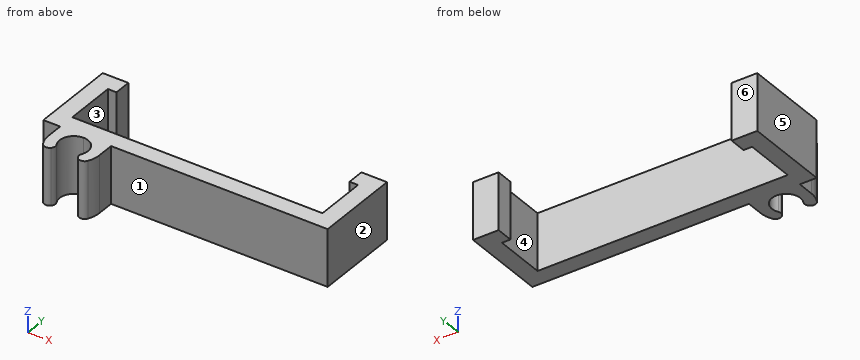
```python
from build123d import *

# Parameters (mm, degrees)
F1_DEPTH    = 10
F2_T1_DEPTH = 16.5073043021
F2_T3_DEPTH = 14.2705098312


# Not quite as in the source:
# - a fillet or chamfer that OpenCascade refuses, or shapes differently, is made with other operations: its cross-section is extruded or revolved along the edge and cut away or added


with BuildPart() as f1:
    # F0 (on Top) → F1 (new body)
    with BuildSketch(Plane.XY):
        with BuildLine():
            Line((-25.6786430255, 0), (12.4131741374, 0))
            Line((12.4131741374, 0), (12.4131741374, 15))
            Line((12.4131741374, 15), (7.9131741374, 15))
            Line((7.9131741374, 15), (7.9131741374, 12))
            Line((7.9131741374, 12), (9.4131741374, 12))
            Line((9.4131741374, 12), (9.4131741374, 3))
            Line((9.4131741374, 3), (-34.5868258626, 3))
            Line((-34.5868258626, 3), (-34.5868258626, 12))
            Line((-34.5868258626, 12), (-33.0868258626, 12))
            Line((-33.0868258626, 12), (-33.0868258626, 15))
            Line((-33.0868258626, 15), (-37.5868258626, 15))
            Line((-37.5868258626, 15), (-37.5868258626, 0))
            Line((-37.5868258626, 0), (-34.6318436787, 0))
            Line((-34.6318436787, 0), (-34.6318436787, -2.9766003136))
            ThreePointArc((-34.6318436787, -2.9766003136), (-34.291082769, -4.6897210919), (-33.3206777997, -6.1420347612))
            Line((-33.3206777997, -6.1420347612), (-31.923010305, -4.7443672665))
            ThreePointArc((-31.923010305, -4.7443672665), (-32.4649421833, -2.0198917326), (-30.1552433521, -0.4766003136))
            ThreePointArc((-30.1552433521, -0.4766003136), (-27.8455445208, -2.0198917326), (-28.3874763991, -4.7443672665))
            Line((-28.3874763991, -4.7443672665), (-26.9898089045, -6.1420347612))
            ThreePointArc((-26.9898089045, -6.1420347612), (-26.0194039351, -4.6897210919), (-25.6786430255, -2.9766003136))
            Line((-25.6786430255, -2.9766003136), (-25.6786430255, 0))
        make_face()
    extrude(amount=F1_DEPTH)

    # F2: fillet of radius 1 on 4 edges, made by hand

    # F2_s2 → F2_t1 (cut)
    with BuildSketch(Plane.XY.offset(-3.253652151)):
        with BuildLine():
            ThreePointArc((-32.5096806342, -5.3310375957), (-33.3621500528, -5.6133092576), (-34.0974017442, -5.0977645446))
            ThreePointArc((-34.0974017442, -5.0977645446), (-33.7471918574, -5.6482770191), (-33.3206777997, -6.1420347612))
            Line((-33.3206777997, -6.1420347612), (-32.5096806342, -5.3310375957))
        make_face()
        with BuildLine():
            ThreePointArc((-27.8008060699, -5.3310375957), (-26.9483366513, -5.6133092576), (-26.2130849599, -5.0977645446))
            ThreePointArc((-26.2130849599, -5.0977645446), (-26.5632948467, -5.6482770191), (-26.9898089045, -6.1420347612))
            Line((-26.9898089045, -6.1420347612), (-27.8008060699, -5.3310375957))
        make_face()
    extrude(amount=F2_T1_DEPTH, mode=Mode.SUBTRACT)

    # F2_s4 → F2_t3 (cut)
    with BuildSketch(Plane.XY.offset(-2.1352549156)):
        with BuildLine():
            ThreePointArc((-32.5269515972, -5.3483085587), (-32.2445345415, -4.7855713596), (-32.3543969423, -4.1656013592))
            ThreePointArc((-32.3543969423, -4.1656013592), (-32.1597026664, -4.4706360752), (-31.923010305, -4.7443672665))
            Line((-31.923010305, -4.7443672665), (-32.5269515972, -5.3483085587))
        make_face()
        with BuildLine():
            ThreePointArc((-27.9560897618, -4.1656013592), (-28.0659521626, -4.7855713596), (-27.7835351069, -5.3483085587))
            Line((-27.7835351069, -5.3483085587), (-28.3874763991, -4.7443672665))
            ThreePointArc((-28.3874763991, -4.7443672665), (-28.1507840377, -4.4706360752), (-27.9560897618, -4.1656013592))
        make_face()
    extrude(amount=F2_T3_DEPTH, mode=Mode.SUBTRACT)


solid = f1.part
```
The listing builds one solid part. Answer for the finished solid, in the listing's coordinates (mm). Face numbers are marked on the shaded views. A direction names the side the tool comes from. Coordinates: 2 decimals unless noted, no trailing zeros. Write each loop counter-clockwise with the first axis right and the second up, starting at its lowest first coordinate (ties: lowest second). Pieces come first, ordered by that corner, then holes. Notation, with made-up numbers: (51.25, 84) - (74.25, 84) arc R9 ccw to (74.25, 99) - close; hole circle Ø2 at (61, 0). An arc over 180 degrees is marked (long way). Return JSON: item names as keys, results as strings. Group by question number.
Q1. The part is cut by section B-B on y = 9.5. Write down the section's boundary in (x, z).
Q2. Which of the six approach directions +Z, -Z, +X, -X, +Y, -Y give full straight-line access (tool end or side, diameter ignored) to the marked faces 1 and 2?
Q3. The part is cut by section D-D on x = 2. Write down the section's boundary in (y, z).
Q4. The part is cut by section C-C on z = 2.75. Write down the section's boundary in (x, y), and give its area (3 significant figures).
Q5. For a pull along Y with two mould halves and no side action, classify the marked faces 3, 4, 5 and 6 as +Y half, -Y half, draft (parallel to the pull), parting line (faces both ways), or undercut.
Q6. The part is cut by section A-A on y = 13.5. Write down the section's boundary in (x, z).
Q7. Flat-ended cylindrical pins translate along their axes: pin 1 Ø6 at (x, y) = (-2.5, 2) entering from -Z; pin 2 Ø3 at (x, z) = (-20.5, 4) entering from +Y; pin 3 Ø5 at (x, y) = (-28.5, 11.5) entering from +Z; pin 4 Ø0.9 at (y, z) = (-1.5, 6) entering from +X. Find the tip coordinate at first contact, or state that the pin passes through.
Q8. Find the intervals of material crossed by line 1 along X through (y, z) = (8.25, 3.5); line 2 along X through (y, z) = (13.5, 8); line 3 along Y through (x, z) = (-5, 5.5), in increasing order. Write a range as [from, to].
Evaluation:
{
 "1": {"outline": "(-37.59, 0) - (-34.59, 0) - (-34.59, 10) - (-37.59, 10) - close; (9.41, 0) - (12.41, 0) - (12.41, 10) - (9.41, 10) - close"},
 "2": {"face 1": "+Z, -Z, +X, -Y", "face 2": "+Z, -Z, +X, +Y, -Y"},
 "3": {"outline": "(0, 0) - (3, 0) - (3, 10) - (0, 10) - close"},
 "4": {"outline": "(-37.59, 0) - (-34.63, 0) - (-34.63, -2.98) arc R4.48 ccw to (-34.1, -5.1) arc R1 ccw to (-32.52, -5.34) arc R1 ccw to (-32.35, -4.17) arc R2.5 cw (long way) to (-27.96, -4.17) arc R1 ccw to (-27.79, -5.34) arc R1 ccw to (-26.21, -5.1) arc R4.48 ccw to (-25.68, -2.98) - (-25.68, 0) - (12.41, 0) - (12.41, 15) - (7.91, 15) - (7.91, 12) - (9.41, 12) - (9.41, 3) - (-34.59, 3) - (-34.59, 12) - (-33.09, 12) - (-33.09, 15) - (-37.59, 15) - close", "area": "258 mm2"},
 "5": {"face 3": "undercut", "face 4": "undercut", "face 5": "draft", "face 6": "+Y half"},
 "6": {"outline": "(-37.59, 0) - (-33.09, 0) - (-33.09, 10) - (-37.59, 10) - close; (7.91, 0) - (12.41, 0) - (12.41, 10) - (7.91, 10) - close"},
 "7": {"pin 1": "stops at z = 0", "pin 2": "stops at y = 3", "pin 3": "passes through", "pin 4": "stops at x = -25.68"},
 "8": {"line 1": "x = [-37.59, -34.59], [9.41, 12.41]", "line 2": "x = [-37.59, -33.09], [7.91, 12.41]", "line 3": "y = [0, 3]"}
}
